The figure shows three views and two pictorial views of one solid part (mm, origin at its lowest corner). Answer the questions. Coordinates: 2 decimals unless noted, no trailing zeros. Order: outer loops, then holes, each group sorted by start corner. A loop starts at its lowest first (then second) coordinate and runs counter-clockwise, first axis right, second up.
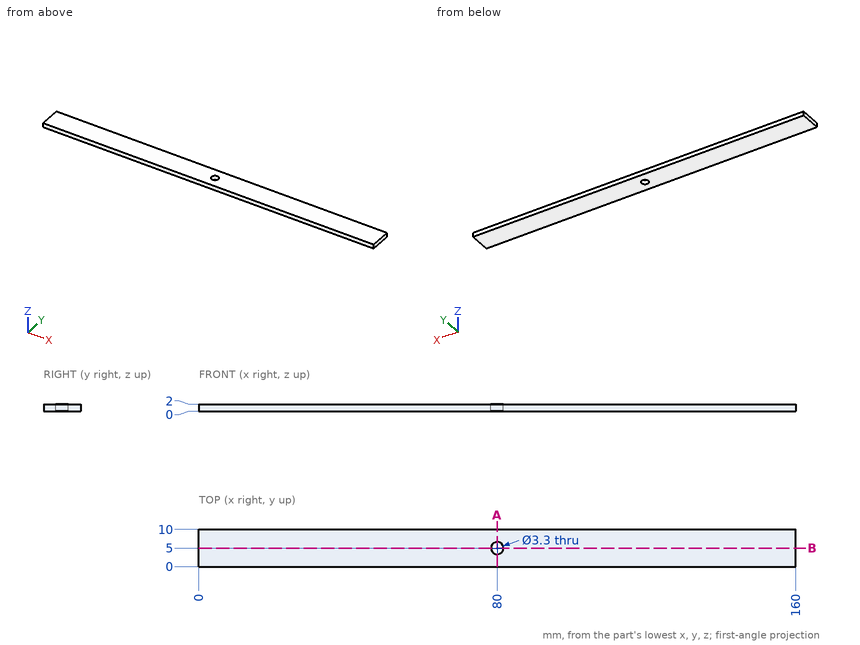
1) A cutting plane is placed at B-B, the plane y = 5. Write down the section's boundary in (x, z), plus the area to 3 significant figures.
2) A cutting plane is placed at A-A, the plane x = 80. Write down the section's boundary in (y, z).
3) Straight lines are drawn through the part: probe 1 along Y at (x, z) = (80, 1.2); probe 2 along X at (y, z) = (4.75, 0.6); probe 3 along X at (y, z) = (3.5, 1.8). For each, find the intervals that lie inside material, in ascending order.
Working result:
1. outline: (0, 0) - (78.35, 0) - (78.35, 2) - (0, 2) - close; (81.65, 0) - (160, 0) - (160, 2) - (81.65, 2) - close
1. area: 313 mm2
2. outline: (0, 0) - (3.35, 0) - (3.35, 2) - (0, 2) - close; (6.65, 0) - (10, 0) - (10, 2) - (6.65, 2) - close
3. probe 1: y = 0 to 3.35, 6.65 to 10
3. probe 2: x = 0 to 78.37, 81.63 to 160
3. probe 3: x = 0 to 79.31, 80.69 to 160
